```python
from build123d import *

# Parameters (mm, degrees)
F1_W     = 9.3304801267
F1_H     = 7.7842138708
F1_W_2   = 7.8273694962
F1_H_2   = 7.4135381728
F1_W_3   = 29.2622358538
F1_H_3   = 7.2785243392
F1_W_4   = 7.6639167964
F1_H_4   = 5.8850795031
F1_H_5   = 10.659635067
F2_DEPTH = 7


# Not quite as in the source:
# - a feature names something its author has since deleted; it is built from what else it names


with BuildPart() as f2:
    # F1 (on Top) → F2 (new body)
    with BuildSketch(Plane.XY):
        Polygon((-41.9203750789, 47.4954210222), (-41.9203750789, 16.0942748189), (-3.3160478342, 16.0942748189), (-3.3160478342, 27.0578376949), (-14.6702602506, 27.0578376949), (-14.6702602506, 34.84358266), (-3.3160478342, 34.84358266), (-3.3160478342, 47.4954210222), (-14.6702602506, 47.4954210222), (-14.6702602506, 57.5520098209), (0, 57.5520098209), (0, 16.0942748189), (27.8269369155, 16.0942748189), (27.8269369155, 18.2988718152), (27.8269369155, 27.0578376949), (13.8774756342, 27.0578376949), (13.8774756342, 57.5520098209), (27.8269369155, 57.5520098209), (27.8269369155, 71.1770653725), (27.4223256856, 71.1770653725), (19.7584088892, 71.1770653725), (11.9310393929, 71.1770653725), (11.9310393929, 87.7217799425), (0, 87.7217799425), (0, 71.1770653725), (-6.0202269815, 71.1770653725), (-35.2824628353, 71.1770653725), (-42.8935922682, 71.1770653725), (-42.8935922682, 57.5520098209), (-28.6197233945, 57.5520098209), (-28.6197233945, 27.0578376949), (-32.1881920099, 27.0578376949), (-32.1881920099, 47.4954210222), align=None)
        Polygon((-3.3160478342, 16.0942748189), (-41.9203750789, 16.0942748189), (-41.9203750789, 0), (-3.3160478342, 0), (-3.3160478342, 12.5654535368), align=None)
        Polygon((-3.3160478342, 27.0578376949), (-3.3160478342, 16.0942748189), (-3.3160478342, 12.5654535368), (11.9310393929, 12.5654535368), (11.9310393929, -2.6322980411), (27.8269369155, -2.6322980411), (27.8269369155, 16.0942748189), (0, 16.0942748189), (0, 57.5520098209), (-14.6702602506, 57.5520098209), (-14.6702602506, 47.4954210222), (-3.3160478342, 47.4954210222), (-3.3160478342, 34.84358266), (-14.6702602506, 34.84358266), (-14.6702602506, 27.0578376949), align=None)
        Polygon((-3.3160478342, 0), (-41.9203750789, 0), (-56.0475625098, 0), (-56.0475625098, -17.8618896753), (-35.2824628353, -17.8618896753), (-56.0475625098, -38.2491163909), (-53.4528233111, -49.7401021421), (-41.7488545561, -38.2491163909), (-41.7488545561, -69.7566494346), (-30.4708592594, -66.4205625653), (-27.8442800045, -41.9240482152), (-23.0254810303, -56.7511208355), (-6.3450210728, -56.7511208355), (-3.3160478342, -108.2752048969), (11.9310393929, -93.3055765817), (11.9310393929, -57.1217983961), (32.2053730488, -57.1217983961), (32.2053730488, -2.6322980411), (27.8269369155, -2.6322980411), (11.9310393929, -2.6322980411), (11.9310393929, 12.5654535368), (-3.3160478342, 12.5654535368), align=None)
        Polygon((-12.6465279609, -38.2491163909), (-12.6465279609, -34.5105081797), (-12.6465279609, -33.1628471613), (-2.621053718, -33.1628471613), (-2.621053718, -41.9242307544), (-12.6465279609, -41.9242307544), align=None, mode=Mode.SUBTRACT)
        with Locations((-7.9812878976, -18.7567416579)):
            Rectangle(F1_W, F1_H, mode=Mode.SUBTRACT)
        Polygon((11.9310393929, -41.9240482152), (11.9310393929, -38.2491163909), (11.9310393929, -34.5105081797), (19.2130599171, -34.5105081797), (19.2130599171, -41.9973358512), (11.9310393929, -41.9973358512), align=None, mode=Mode.SUBTRACT)
        with Locations((15.8447241411, -18.5714038089)):
            Rectangle(F1_W_2, F1_H_2, mode=Mode.SUBTRACT)
        with Locations((-20.6513449084, 74.8163275421)):
            Rectangle(F1_W_3, F1_H_3)
        Polygon((-35.6308221817, 88.9063850045), (-35.2824628353, 78.4555897117), (-6.0202269815, 78.4555897117), (-6.0202269815, 88.9063850045), align=None)
        with Locations((23.5903672874, 74.119605124)):
            Rectangle(F1_W_4, F1_H_4)
        with Locations((23.5903672874, 82.391962409)):
            Rectangle(F1_W_4, F1_H_5)
    extrude(amount=F2_DEPTH)


solid = f2.part
```
Build history of the part. All positions in model axes, mm. A direction names the side the tool comes from. Round coordinates to 2 decimals unless told otherwise and drop trailing zeros. Write each loop counter-clockwise with the first axis right and the second up, starting at its lowest first coordinate (ties: lowest second). Pieces come first, ordered by that corner, then holes. Notation, with made-up numbers: (80, 83.25) - (92, 83.25) arc R15 ccw to (92, 109.25) - close; hole circle Ø5 at (70, -36). An arc over 180 degrees is marked (long way). Write each question's results on one line, items separated by ' | '. Start each with the question number.
Item 1: Which spindle directions (+Z, -Z, +X, -X, +Y, -Y) get a long thin tool onto all of the face, cutting with end or side? Do faces 4 (the face through (21, 27.058, 3)), 5 (the face through (-8, -14.865, 3)), 6 (the face through (-37, 47.495, 3)), 7 (the face through (-4.85, -82.15, 3.45)). Say none if no direction does.
Item 2: Wall check: L1, parallel to Y at x = 16.5, z = 4.5; L2, parallel to X at y = 30.5, z = 4; L3, parallel to Y at x = 13, z = 4. Give the ranges that are in metal, low to high. Write a range as [from, to].
Item 3: Saw through at C-C (x = -16.5). Write the cut outline in (y, z).
Item 4: Saw through at B-B (y = 60.5). Write the cut outline in (x, z).
Item 5: Saw through at A-A (z = 2.25). State how many separate pieces and enclosed holes the cut face has, and give its area (3 significant figures).
Item 6: Mould opens along Y. For faces 1 (the face through (16, 71.177, 3)), 2 (the face through (27.827, 64, 3)), 3 (the face through (-2.621, -37, 3)) say: pulls with the +Y half, pulls with the -Y half, needs draft (parallel to the pull), parting line crosses it, or undercut.
Item 7: Drop flat-ended pins along their axis: P1, Ø8, axis at x = 16.5, y = 55.5, coming from the +Z side; P2, Ø3.5, axis at y = 78.5, z = 2.5, coming from the -X side; P3, Ø2, axis at y = 80, z = 2.5, coming from the +X side; P4, Ø1.5, axis at y = -22.5, z = 1, coming from the -X side. Give the stop position or say it passes through.
Results are:
1) face 4: +Z, -Z, +X | face 5: +Z, -Z | face 6: +Z, -Z, -X | face 7: +Z, -Z, -Y
2) L1: y = [-57.12, -42], [-34.51, -22.28], [-14.86, 27.06], [57.55, 71.18] | L2: x = [-41.92, -32.19], [-28.62, 13.88] | L3: y = [-57.12, -42], [-34.51, -22.28], [-14.86, 71.18]
3) outline: (-56.75, 0) - (88.91, 0) - (88.91, 7) - (-56.75, 7) - close
4) outline: (-42.89, 0) - (27.83, 0) - (27.83, 7) - (-42.89, 7) - close
5) separate pieces: 1 | enclosed holes: 4 | area: 10,400 mm²
6) face 1: pulls with the +Y half | face 2: needs draft | face 3: undercut
7) P1: stops at z = 7 | P2: stops at x = -35.34 | P3: stops at x = 27.42 | P4: stops at x = -40.77
